```python
from build123d import *

# Parameters (mm, degrees)
SKETCH1_W                 = 407
SKETCH1_H                 = 788
BOSS_EXTRUDE1_DEPTH       = 10
SHELL1_T                  = -1.5
SKETCH2_W                 = 80
SKETCH2_H                 = 80
BOSS_EXTRUDE2_DEPTH       = 4
SKETCH3_R                 = 35
CUT_EXTRUDE1_DEPTH        = 3
BOSS_EXTRUDE3_DEPTH       = 15
SKETCH5_R                 = 5.284188489
BOSS_EXTRUDE4_DEPTH       = 2
FILLET1_R                 = 3
FILLET2_R                 = 1
SKETCH6_W                 = 5.396205122
SKETCH6_H                 = 1.259856044
CUT_EXTRUDE2_DEPTH        = 5
BOSS_EXTRUDE5_START       = -71.5
SKETCH7_R                 = 6
SKETCH7_R_2               = 2
BOSS_EXTRUDE5_DEPTH       = 12.5
MIRROR2_START             = -71.5
MIRROR2_COPY_1_SKETCH_R   = 6
MIRROR2_COPY_1_SKETCH_R_2 = 2
MIRROR2_COPY_1_DEPTH      = 12.5


with BuildPart() as part:
    # Sketch1 → Boss-Extrude1 (new, symmetric)
    with BuildSketch(Plane.XY):
        Rectangle(SKETCH1_W, SKETCH1_H)
    extrude(amount=BOSS_EXTRUDE1_DEPTH, both=True)

    # Shell1
    shell1_openings = [part.faces().sort_by_distance(p)[0] for p in [
        (0, 0, -10),
    ]]
    offset(amount=SHELL1_T, openings=shell1_openings, kind=Kind.INTERSECTION)

    # Sketch2 → Boss-Extrude2 (add)
    with BuildSketch(Plane.XY.offset(10)):
        with Locations((128.5, 0)):
            Rectangle(SKETCH2_W, SKETCH2_H)
    extrude(amount=BOSS_EXTRUDE2_DEPTH)

    # Sketch3 → Cut-Extrude1 (cut)
    with BuildSketch(Plane.XY.offset(14)):
        with Locations((128.5, 0)):
            Circle(SKETCH3_R)
    extrude(amount=-CUT_EXTRUDE1_DEPTH, mode=Mode.SUBTRACT)

    # Sketch4 → Boss-Extrude3 (add)
    with BuildSketch(Plane.XY.offset(11)):
        with BuildLine():
            ThreePointArc((139.828046269, 11.018836293), (128.5, 28.547480442), (117.171953731, 11.018836293))
            ThreePointArc((117.171953731, 11.018836293), (119.53963249, 0), (117.171953731, -11.018836293))
            ThreePointArc((117.171953731, -11.018836293), (128.5, -28.547480442), (139.828046269, -11.018836293))
            ThreePointArc((139.828046269, -11.018836293), (137.46036751, 0), (139.828046269, 11.018836293))
        make_face()
    extrude(amount=BOSS_EXTRUDE3_DEPTH)

    # Sketch5 → Boss-Extrude4 (add)
    with BuildSketch(Plane.XY.offset(26)):
        with Locations((128.5, 16.12273172)):
            Circle(SKETCH5_R)
    extrude(amount=BOSS_EXTRUDE4_DEPTH)

    # Fillet1
    fillet1_edges = [part.edges().sort_by_distance(p)[0] for p in [
        (137.46036751, 0, 26),
        (128.5, 28.547480442, 26),
        (119.53963249, 0, 26),
        (128.5, -28.547480442, 26),
    ]]
    fillet(fillet1_edges, radius=FILLET1_R)

    # Fillet2
    fillet2_edges = [part.edges().sort_by_distance(p)[0] for p in [
        (123.215811511, 16.12273172, 28),
    ]]
    fillet(fillet2_edges, radius=FILLET2_R)

    # Sketch6 → Cut-Extrude2 (cut)
    with BuildSketch(Plane.XY.offset(28)):
        with Locations((128.5, 16.12273172)):
            Rectangle(SKETCH6_W, SKETCH6_H)
    extrude(amount=-CUT_EXTRUDE2_DEPTH, mode=Mode.SUBTRACT)

    # Sketch7 → Boss-Extrude5 (add)
    with BuildSketch(Plane(origin=(0, 394, 0), x_dir=(1, 0, 0), z_dir=(0, 1, 0)).offset(BOSS_EXTRUDE5_START)):
        with Locations((-193.5, -3)):
            Circle(SKETCH7_R)
        with Locations(Location((-193.5, -3, 0), (0, 0, 270))):
            Circle(SKETCH7_R_2, mode=Mode.SUBTRACT)
    boss_extrude5 = extrude(amount=-BOSS_EXTRUDE5_DEPTH)

    # Mirror1: Boss-Extrude5 across plane
    add(boss_extrude5.mirror(Plane(origin=(0, 292, 0), x_dir=(0, 0, 1), z_dir=(0, -1, 0))))

    # Mirror2: Boss-Extrude5 across plane
    add(boss_extrude5.mirror(Plane.ZX))

    # Mirror2 copy 1 sketch → Mirror2 copy 1 (add)
    with BuildSketch(Plane(origin=(0, -190, 0), x_dir=(1, 0, 0), z_dir=(0, 1, 0)).offset(MIRROR2_START)):
        with Locations((-193.5, -3)):
            Circle(MIRROR2_COPY_1_SKETCH_R)
        with Locations(Location((-193.5, -3, 0), (0, 0, 270))):
            Circle(MIRROR2_COPY_1_SKETCH_R_2, mode=Mode.SUBTRACT)
    extrude(amount=-MIRROR2_COPY_1_DEPTH)


solid = part.part
```
Source: CAD feature listing. Evaluate the final solid. Frame: model axes, mm. A direction names the side the tool comes from. Coordinates: 2 decimals unless noted, no trailing zeros. Order: outer loops, then holes, each group sorted by start corner. A loop starts at its lowest first (then second) coordinate and runs counter-clockwise, first axis right, second up. Notation, with made-up numbers: M 32.25,21.5 L 44.25,21.5 A19 ccw 44.25,26.5 Z; hole C -22,65.25 d7. An arc over 180 degrees is marked long. Write each question's results on one line, items separated by ' | '. Start each with the question number.
1) Line query: line 1 (X direction, y = -271, z = 3); line 2 (X direction, y = 128, z = -3); line 3 (Z direction, x = -193, y = -269). Output: solid intervals per line, ascending. Write a range as from..to.
2) Access query for faces 4 (the face through (-3, 394, 0)), 5 (the face through (128.847, 28.543, 16.916)), 6 (the face through (-3, 392.5, -1)). Directions: +Z, -Z, +X, -X, +Y, -Y. A direction counts if a zero-diameter tool reaches every point of the face in a straight line with its end or side. Return the directions, or none.
3) Draft query along Y for faces 1 (the face through (-3, 6, 10)), 2 (the face through (202, -5, -1)), 3 (the face through (-3, -394, 0)). Return one class per face: released by +Y, released by -Y, zero draft, split by the parting line, or undercut.
4) Section query A-A (y = 0). Return the cut outline in (x, z), plus the area to 3 significant figures.
5) Section query B-B (x = -37). Return the cut outline in (y, z), plus the area to 3 significant figures.
6) Contact query for flat-ended pins moving along their axis: pin 1 Ø1.5 at (x, y) = (-37.5, 220.5) entering from +Z; pin 2 Ø4.5 at (y, z) = (-11.5, 11) entering from -X; pin 3 Ø4 at (x, z) = (127.5, 25) entering from -Y; pin 4 Ø2 at (x, y) = (73.5, -85.5) entering from -Z. Output: stop coordinate, or through.
7) Section query C-C (y = 121). Return the cut outline in (x, z).
Answers:
1) line 1: x = -203.5..-202, -199.5..-195.5, -191.5..-187.5, 202..203.5 | line 2: x = -203.5..-202, 202..203.5 | line 3: z = -2.98..1.06, 4.94..10
2) face 4: +Z, -Z, +X, -X, +Y | face 5: +Z | face 6: -Z
3) face 1: zero draft | face 2: undercut | face 3: released by -Y
4) outline: M -203.5,-10 L -202,-10 L -202,8.5 L 202,8.5 L 202,-10 L 203.5,-10 L 203.5,10 L 168.5,10 L 168.5,14 L 163.5,14 L 163.5,11 L 137.46,11 L 137.46,23 A3 ccw 134.46,26 L 122.54,26 A3 ccw 119.54,23 L 119.54,11 L 93.5,11 L 93.5,14 L 88.5,14 L 88.5,10 L -203.5,10 Z | area: 1,040 mm^2
5) outline: M -394,-10 L -392.5,-10 L -392.5,8.5 L 392.5,8.5 L 392.5,-10 L 394,-10 L 394,10 L -394,10 Z | area: 1,240 mm^2
6) pin 1: stops at z = 10 | pin 2: stops at x = -203.5 | pin 3: stops at y = -28.54 | pin 4: stops at z = 8.5
7) outline: M -203.5,-10 L -202,-10 L -202,8.5 L 202,8.5 L 202,-10 L 203.5,-10 L 203.5,10 L -203.5,10 Z
